from build123d import *

# Parameters (mm, degrees)
ESQUISSE1_W             = 18
ESQUISSE1_H             = 29
BOSS_EXTRU_1_DEPTH      = 46.2
ESQUISSE3_R             = 1
ENL_V_MAT_EXTRU_1_DEPTH = 58.440752084
ESQUISSE4_W             = 18
ESQUISSE4_H             = 30
ENL_V_MAT_EXTRU_2_DEPTH = 58.440752084
ESQUISSE5_W             = 8.1
ESQUISSE5_H             = 46.2
BOSS_EXTRU_2_DEPTH      = 29
CONG_1_R                = 3.5
ENL_V_START             = -46.2
ESQUISSE7_W             = 18
ESQUISSE7_H             = 18
ENL_V_MAT_EXTRU_4_DEPTH = 46.2
ESQUISSE8_W             = 15
ESQUISSE8_H             = 46.2
ESQUISSE8_R             = 2.25
BOSS_EXTRU_3_DEPTH      = 11
CHANFREIN1_SIZE         = 9
CONG_2_R                = 3.5


with BuildPart() as part:
    # Esquisse1 → Boss.-Extru.1 (new body)
    with BuildSketch(Plane.XY):
        with Locations((9, 14.5)):
            Rectangle(ESQUISSE1_W, ESQUISSE1_H)
    extrude(amount=BOSS_EXTRU_1_DEPTH)

    # Esquisse3 → Enl_v. mat.-Extru.1 (cut, through all)
    with BuildSketch(Plane.XY.offset(46.2)):
        with Locations((2.5, 26.2)):
            Circle(ESQUISSE3_R)
        with Locations((2.5, 9.2)):
            Circle(ESQUISSE3_R)
    extrude(amount=-ENL_V_MAT_EXTRU_1_DEPTH, mode=Mode.SUBTRACT)

    # Esquisse4 → Enl_v. mat.-Extru.2 (cut, through all)
    with BuildSketch(Plane(origin=(0, 29, 0), x_dir=(1, 0, 0), z_dir=(0, 1, 0))):
        with Locations((9, -23.1)):
            Rectangle(ESQUISSE4_W, ESQUISSE4_H)
    extrude(amount=-ENL_V_MAT_EXTRU_2_DEPTH, mode=Mode.SUBTRACT)


with BuildPart() as enl_v_mat_extru_2_piece_1:
    # of the separate pieces the step leaves, piece 1, a body of its own (enl_v_mat_extru_2_pieces)
    add(part.part.solids().sort_by_distance((0, 0, 0))[0])



with BuildPart() as enl_v_mat_extru_2_piece_2:
    # of the separate pieces the step leaves, piece 2, a body of its own (enl_v_mat_extru_2_pieces)
    add(part.part.solids().sort_by_distance((18, 0, 38.1))[0])


with BuildPart() as enl_v_mat_extru_2_piece_1_1:
    add(enl_v_mat_extru_2_piece_1.part)

    add(enl_v_mat_extru_2_piece_2.part)  # Boss.-Extru.2 merges Enl_v. mat.-Extru.2 piece 2
    # Esquisse5 → Boss.-Extru.2 (add)
    with BuildSketch(Plane(origin=(0, 29, 0), x_dir=(1, 0, 0), z_dir=(0, 1, 0))):
        with Locations((22.05, -23.1)):
            Rectangle(ESQUISSE5_W, ESQUISSE5_H)
    extrude(amount=-BOSS_EXTRU_2_DEPTH)

    # Cong_1
    cong_1_edges = [enl_v_mat_extru_2_piece_1_1.edges().sort_by_distance(p)[0] for p in [
        (0, 29, 42.15),
        (0, 29, 4.05),
    ]]
    fillet(cong_1_edges, radius=CONG_1_R)

    # Esquisse7 → Enl_v. mat.-Extru.4 (cut)
    with BuildSketch(Plane(origin=(0, 0, 0), x_dir=(-1, 0, 0), z_dir=(0, 0, -1)).offset(ENL_V_START)):
        with Locations((-17.1, 20)):
            Rectangle(ESQUISSE7_W, ESQUISSE7_H)
    extrude(amount=ENL_V_MAT_EXTRU_4_DEPTH, mode=Mode.SUBTRACT)

    # Esquisse8 → Boss.-Extru.3 (add)
    with BuildSketch(Plane(origin=(0, 11, 0), x_dir=(1, 0, 0), z_dir=(0, 1, 0))):
        with Locations((33.6, -23.1)):
            Rectangle(ESQUISSE8_W, ESQUISSE8_H)
        with Locations(Location((33.6, -5.5, 0), (0, 0, 270))):
            Circle(ESQUISSE8_R, mode=Mode.SUBTRACT)
        with Locations(Location((33.6, -32.5, 0), (0, 0, 270))):
            Circle(ESQUISSE8_R, mode=Mode.SUBTRACT)
        with Locations(Location((33.6, -19, 0), (0, 0, 270))):
            Circle(ESQUISSE8_R, mode=Mode.SUBTRACT)
    extrude(amount=-BOSS_EXTRU_3_DEPTH)

    # Chanfrein1
    chanfrein1_edges = [enl_v_mat_extru_2_piece_1_1.edges().sort_by_distance(p)[0] for p in [
        (8.1, 11, 42.15),
        (8.1, 11, 4.05),
    ]]
    chamfer(chanfrein1_edges, length=CHANFREIN1_SIZE)

    # Cong_2
    cong_2_edges = [enl_v_mat_extru_2_piece_1_1.edges().sort_by_distance(p)[0] for p in [
        (8.1, 29, 42.15),
        (8.1, 29, 4.05),
    ]]
    fillet(cong_2_edges, radius=CONG_2_R)


solid = enl_v_mat_extru_2_piece_1_1.part
Geometry check sheet. Reference: the model listing, model coordinates, mm. A direction names the side the tool comes from. Round coordinates to 2 decimals unless told otherwise and drop trailing zeros. Loops run counter-clockwise (first coordinate to the right, second up) from the corner with the lowest first, then second, coordinate; pieces in that order, holes last. Notation, with made-up numbers: (77.5, -30) - (93.5, -30) arc R27 ccw to (93.5, -4) - close; hole circle Ø6 at (76.5, 9). An arc over 180 degrees is marked (long way). Answer as CSV lines item,"result".
(1) Release check for a two-part mould opening along X. For faces 1 (the face through (16, 8, 46.2)), 2 (the face through (1, 27.95, 42.21)), 3 (the face through (7.1, 27.95, 3.99)), 4 (the face through (35.497, 5.577, 6.71)) record: released by +X, released by -X, zero draft, split by the parting line, or undercut.
Output values:
face 1,"zero draft"
face 2,"released by -X"
face 3,"released by +X"
face 4,"undercut"
(2) Cross-section at C-C, the plane x = 12.5. Enter the section's corners in (y, z).
Output values:
outline,"(0, 0) - (15.6, 0) - (15.6, 8.1) - (0, 8.1) - close; (0, 38.1) - (15.6, 38.1) - (15.6, 46.2) - (0, 46.2) - close"
(3) Cross-section at A-A, the plane z = 5.5. Enter the section's corners in (x, y).
Output values:
outline,"(0, 0) - (31.35, 0) - (31.35, 11) - (17.1, 11) - (8.1, 20) - (8.1, 25.5) arc R3.5 ccw to (4.6, 29) - (3.5, 29) arc R3.5 ccw to (0, 25.5) - close; (35.85, 0) - (41.1, 0) - (41.1, 11) - (35.85, 11) - close; hole circle Ø2 at (2.5, 9.2); hole circle Ø2 at (2.5, 26.2)"
(4) Material ranges on line 1 along Z through (x, y) = (5.5, 16.25); line 2 along X through (y, z) = (4, 19); line 3 along Y through (x, z) = (2.5, 2), recorded low to high.
Output values:
line 1,"z = 0 to 8.1, 38.1 to 46.2"
line 2,"x = 18 to 31.35, 35.85 to 41.1"
line 3,"y = 0 to 8.2, 10.2 to 25.2, 27.2 to 28.85"
(5) Cross-section at B-B, the plane x = 33.6. Enter the section's corners in (y, z).
Output values:
outline,"(0, 0) - (11, 0) - (11, 3.25) - (0, 3.25) - close; (0, 7.75) - (11, 7.75) - (11, 16.75) - (0, 16.75) - close; (0, 21.25) - (11, 21.25) - (11, 30.25) - (0, 30.25) - close; (0, 34.75) - (11, 34.75) - (11, 46.2) - (0, 46.2) - close"
(6) Cross-section at D-D, the plane y = 9.2. Enter the section's corners in (x, z), and give its area (3 significant figures).
Output values:
outline,"(0, 0) - (1.5, 0) - (1.5, 8.1) - (0, 8.1) - close; (0, 38.1) - (1.5, 38.1) - (1.5, 46.2) - (0, 46.2) - close; (3.5, 0) - (41.1, 0) - (41.1, 46.2) - (3.5, 46.2) - (3.5, 38.1) - (18, 38.1) - (18, 8.1) - (3.5, 8.1) - close; hole circle Ø4.5 at (33.6, 5.5); hole circle Ø4.5 at (33.6, 19); hole circle Ø4.5 at (33.6, 32.5)"
area,"1,280 mm²"
(7) Depth check by flat-ended pin: pin 1 Ø6 at (y, z) = (24, 5.5) entering from +X; pin 2 Ø5 at (x, z) = (33.6, 19) entering from +Y; pin 3 Ø3.5 at (y, z) = (8, 18.5) entering from -X. Enter the tip coordinate at first touch or a pass-through.
Output values:
pin 1,"stops at x = 8.1"
pin 2,"stops at y = 11"
pin 3,"stops at x = 18"
(8) Set-up check for faces 5 (the face through (29, 11, 23)), 6 (the face through (7, 11, 8.1)), 7 (the face through (0, 13, 42)): record each of +Z, -Z, +X, -X, +Y, -Y from which the full face is reachable in a straight line by a thin tool's end or side.
Output values:
face 5,"+Z, -Z, +X, +Y"
face 6,"-X, +Y, -Y"
face 7,"+Z, -Z, -X, +Y, -Y"
